from build123d import *

# Parameters (mm, degrees)
F0_R     = 20
F1_DEPTH = 12


with BuildPart() as f1:
    # F0 (on Front) → F1 (new body)
    with BuildSketch(Plane.XZ):
        with BuildLine():
            ThreePointArc((-45.1402234044, 130.0868427911), (-44.3953824054, 132.5425897679), (-44.1438812161, 135.0964551676))
            ThreePointArc((-44.1438812161, 135.0964551676), (-66.902815449, 143.9263254526), (-56.0541389315, 122.0575825878))
            ThreePointArc((-56.0541389315, 122.0575825878), (-49.477735957, 124.5505867663), (-45.1402234044, 130.0868427911))
        make_face()
        with BuildLine():
            ThreePointArc((-45.1402234044, 130.0868427911), (-49.477735957, 124.5505867663), (-56.0541389315, 122.0575825878))
            Line((-56.0541389315, 122.0575825878), (-20.6749169362, 81.5374788645))
            ThreePointArc((-20.6749169362, 81.5374788645), (-15.8403911831, 87.9020164198), (-9.3949234629, 92.6281060737))
            Line((-9.3949234629, 92.6281060737), (-45.1402234044, 130.0868427911))
        make_face()
        with BuildLine():
            ThreePointArc((-9.3949234629, 92.6281060737), (-15.8403911831, 87.9020164198), (-20.6749169362, 81.5374788645))
            ThreePointArc((-20.6749169362, 81.5374788645), (-23.4023159827, 74.4832519056), (-24.1275682376, 66.9549830001))
            ThreePointArc((-24.1275682376, 66.9549830001), (-22.7294741415, 59.3041231282), (-19.2667531461, 52.3399370889))
            ThreePointArc((-19.2667531461, 52.3399370889), (11.8900093443, 41.5257597874), (31.4519924852, 68.0779554628))
            ThreePointArc((31.4519924852, 68.0779554628), (29.653096416, 77.915975697), (24.4892064897, 86.4808405543))
            ThreePointArc((24.4892064897, 86.4808405543), (19.5802695472, 90.8629659463), (13.7789121862, 93.968595935))
            ThreePointArc((13.7789121862, 93.968595935), (2.0453958796, 95.8326850768), (-9.3949234629, 92.6281060737))
        make_face()
        with Locations((3.6508674214, 68.0779554628)):
            Circle(F0_R, mode=Mode.SUBTRACT)
        with BuildLine():
            ThreePointArc((-19.2667531461, 52.3399370889), (-22.7294741415, 59.3041231282), (-24.1275682376, 66.9549830001))
            Line((-24.1275682376, 66.9549830001), (-35.430176559, 66.1910267504))
            ThreePointArc((-35.430176559, 66.1910267504), (-32.4777200289, 63.8186090674), (-30.2460369862, 60.7583875033))
            ThreePointArc((-30.2460369862, 60.7583875033), (-28.9402630028, 57.4278194818), (-28.4958610621, 53.8781383755))
            ThreePointArc((-28.4958610621, 53.8781383755), (-28.5164751814, 53.1079350682), (-28.5782585148, 52.3399370889))
            Line((-28.5782585148, 52.3399370889), (-19.2667531461, 52.3399370889))
        make_face()
        with BuildLine():
            Line((27.3106167301, 102.5154178797), (13.7789121862, 93.968595935))
            ThreePointArc((13.7789121862, 93.968595935), (19.5802695472, 90.8629659463), (24.4892064897, 86.4808405543))
            Line((24.4892064897, 86.4808405543), (40.6466048753, 97.4983605522))
            ThreePointArc((40.6466048753, 97.4983605522), (33.435945257, 98.5644139139), (27.3106167301, 102.5154178797))
        make_face()
        with BuildLine():
            Line((-30.2460369862, 60.7583875033), (-35.430176559, 66.1910267504))
            ThreePointArc((-35.430176559, 66.1910267504), (-55.8007056513, 47.4937303618), (-28.5782585148, 52.3399370889))
            ThreePointArc((-28.5782585148, 52.3399370889), (-28.5164751814, 53.1079350682), (-28.4958610621, 53.8781383755))
            ThreePointArc((-28.4958610621, 53.8781383755), (-28.9402630028, 57.4278194818), (-30.2460369862, 60.7583875033))
        make_face()
        with BuildLine():
            ThreePointArc((-30.2460369862, 60.7583875033), (-32.4777200289, 63.8186090674), (-35.430176559, 66.1910267504))
            Line((-35.430176559, 66.1910267504), (-30.2460369862, 60.7583875033))
        make_face()
        with BuildLine():
            ThreePointArc((56.7421202866, 114.697404157), (32.9131115376, 130.6239087268), (27.3106167301, 102.5154178797))
            ThreePointArc((27.3106167301, 102.5154178797), (33.435945257, 98.5644139139), (40.6466048753, 97.4983605522))
            ThreePointArc((40.6466048753, 97.4983605522), (52.0906202883, 102.9195359578), (56.7421202866, 114.697404157))
        make_face()
    extrude(amount=F1_DEPTH)


solid = f1.part
Verification items for the finished model (mm, model axes). A direction names the side the tool comes from. Round coordinates to 2 decimals unless told otherwise and drop trailing zeros. Loops run counter-clockwise (first coordinate to the right, second up) from the corner with the lowest first, then second, coordinate; pieces in that order, holes last. Notation, with made-up numbers: (45.5, 71) - (83.5, 71) arc R19 cw to (83.5, 105) - close; hole circle Ø3 at (-22, -19.75). An arc over 180 degrees is marked (long way). Use a Markdown table: item, result. Add a question column.
1. Release check for a two-part mould opening along Z. For faces 1 (the face through (2.21, -5.92, 95.84)), 2 (the face through (-56.02, -5.92, 47.96)), 3 (the face through (-12, 0, 90)) record: released by +Z, released by -Z, zero draft, split by the parting line, or undercut.
2. Section check B-B, the plane x = 7. Record the boundary of the cut face in (y, z), plus the area to 3 significant figures.
3. Section check C-C, the plane z = 113. Record the boundary of the cut face in (x, y), plus the area to 3 significant figures.
4. Access from +Z, -Z, +X, -X, +Y, -Y to the whole of each face (thin tool, end or side, straight path). Record for faces 4 (the face through (32.45, -5.92, 91.91)), 5 (the face through (-24, -6, 52.34)), 6 (the face through (20.64, -5.92, 98.3)).
5. Section check D-D, the plane x = 46.5. Record the boundary of the cut face in (y, z).
6. Thickness scan on probe 1 along Z at (x, y) = (-11, -7); probe 2 along X at (y, z) = (-7.75, 59); probe 3 along X at (y, z) = (-6.5, 59.5). Record the ranges inside material, lowest first. Write a range as [from, to].
7. Gauge pin test, flat ends, axial feed: pin 1 (3 mm diameter, centred on y = -10, z = 87.5, fed in from +X); pin 2 (5 mm diameter, centred on y = -6, z = 74, fed in from -X); pin 3 (5 mm diameter, centred on x = -36, y = -8.5, fed in from -Z). Record the tip position at first contact, or that the pin passes through.
8. Section check A-A, the plane y = -5.75. Record the boundary of the cut face in (x, z).
Checks:
| question | item | result |
|---|---|---|
| 1 | face 1 | released by +Z |
| 1 | face 2 | undercut |
| 1 | face 3 | zero draft |
| 2 | outline | (-12, 40.48) - (0, 40.48) - (0, 48.36) - (-12, 48.36) - close; (-12, 87.8) - (0, 87.8) - (0, 95.68) - (-12, 95.68) - close |
| 2 | area | 189 mm^2 |
| 3 | outline | (-48.15, -12) - (-28.83, -12) - (-28.83, 0) - (-48.15, 0) - close; (22.35, -12) - (56.66, -12) - (56.66, 0) - (22.35, 0) - close |
| 3 | area | 643 mm^2 |
| 4 | face 4 | +X, +Y, -Y |
| 4 | face 5 | -Z, +Y, -Y |
| 4 | face 6 | +Y, -Y |
| 5 | outline | (-12, 98.94) - (0, 98.94) - (0, 130.45) - (-12, 130.45) - close |
| 6 | probe 1 | z = [44.45, 54.46], [81.69, 94.31] |
| 6 | probe 2 | x = [-56.35, -14.17], [21.47, 29.93] |
| 6 | probe 3 | x = [-56.15, -14.42], [21.72, 30.1] |
| 7 | pin 1 | stops at x = 28.18 |
| 7 | pin 2 | stops at x = -23.94 |
| 7 | pin 3 | stops at z = 40.17 |
| 8 | outline | (-56.05, 122.06) - (-20.67, 81.54) arc R27.8 ccw to (-24.13, 66.95) - (-35.43, 66.19) arc R14.4 ccw (long way) to (-28.58, 52.34) - (-19.27, 52.34) arc R27.8 ccw (long way) to (24.49, 86.48) - (40.65, 97.5) arc R17.24 ccw (long way) to (27.31, 102.52) - (13.78, 93.97) arc R27.8 ccw to (-9.39, 92.63) - (-45.14, 130.09) arc R13.09 ccw (long way) to start; hole circle Ø40 at (3.65, 68.08) |
